```python
from build123d import *

# Parameters (mm, degrees)
F1_DEPTH = 45
F2_R     = 8.270702783
F2_R_2   = 7.5699344576
F2_R_3   = 0.4069488222
F3_DEPTH = 1.5


with BuildPart() as f1:
    # F0 (on Right) → F1 (new body)
    with BuildSketch(Plane.YZ):
        with BuildLine():
            Line((-22.4725382223, 23.5068366048), (0, 0))
            Line((0, 0), (12.3609593138, 0))
            ThreePointArc((12.3609593138, 0), (13.7751728762, 0.5857864376), (14.3609593138, 2))
            Line((14.3609593138, 2), (14.3609593138, 7))
            Line((14.3609593138, 7), (14.3609593138, 9))
            ThreePointArc((14.3609593138, 9), (14.068066095, 9.7071067812), (13.3609593138, 10))
            Line((13.3609593138, 10), (12.2823521785, 10))
            ThreePointArc((12.2823521785, 10), (11.5752453973, 9.7071067812), (11.2823521785, 9))
            Line((11.2823521785, 9), (11.2823521785, 7))
            ThreePointArc((11.2823521785, 7), (10.1107793032, 4.1715728753), (7.2823521785, 3))
            Line((7.2823521785, 3), (1.2823521785, 3))
            Line((1.2823521785, 3), (-25.4725382223, 30.9862840062))
            ThreePointArc((-25.4725382223, 30.9862840062), (-28.7578385809, 31.6975803479), (-30.6410287362, 28.913206851))
            Line((-30.6410287362, 28.913206851), (-30.6410287362, 0))
            Line((-30.6410287362, 0), (-27.6410287362, 0))
            Line((-27.6410287362, 0), (-27.6410287362, 21.4337594496))
            ThreePointArc((-27.6410287362, 21.4337594496), (-25.7578385809, 24.2181329465), (-22.4725382223, 23.5068366048))
        make_face()
    extrude(amount=F1_DEPTH)

    # F2 (on face) → F3 (cut)
    with BuildSketch(Plane(origin=(0, 2.1684905138, 2.0730771552), x_dir=(-1, 0, 0), z_dir=(0, 0.7228301713, 0.6910257184))):
        with Locations((-22.5, 20.6411760892)):
            Circle(F2_R)
        with Locations((-22.5, 20.6411760892)):
            Circle(F2_R_2, mode=Mode.SUBTRACT)
        with BuildLine():
            Line((-26.7460289363, 19.2989930163), (-26.7460289363, 21.0181410771))
            ThreePointArc((-26.7460289363, 21.0181410771), (-27.1604015057, 23.0993524994), (-27.5180879991, 21.0076531943))
            Line((-27.5180879991, 21.0076531943), (-27.5180879991, 19.1088523712))
            Line((-27.5180879991, 19.1088523712), (-27.3791737854, 18.8299436122))
            Line((-27.3791737854, 18.8299436122), (-27.1837860346, 18.5172446072))
            Line((-27.1837860346, 18.5172446072), (-26.9623473287, 18.2827226818))
            Line((-26.9623473287, 18.2827226818), (-26.68880485, 18.0481951684))
            Line((-26.68880485, 18.0481951684), (-26.3631585985, 17.8918484598))
            Line((-26.3631585985, 17.8918484598), (-25.9333048016, 17.7876148373))
            Line((-25.9333048016, 17.7876148373), (-18.7821220607, 17.7876148373))
            Line((-18.7821220607, 17.7876148373), (-18.5476560146, 17.8918484598))
            Line((-18.5476560146, 17.8918484598), (-18.3392427862, 18.0481951684))
            Line((-18.3392427862, 18.0481951684), (-18.0917512625, 18.2827226818))
            Line((-18.0917512625, 18.2827226818), (-17.9093908519, 18.5172446072))
            Line((-17.9093908519, 18.5172446072), (-17.7009776235, 18.8299436122))
            Line((-17.7009776235, 18.8299436122), (-17.5967700779, 19.1088523712))
            Line((-17.5967700779, 19.1088523712), (-17.5967700779, 21.0005989226))
            ThreePointArc((-17.5967700779, 21.0005989226), (-17.9118361845, 23.10197132), (-18.3392427862, 21.0205400333))
            Line((-18.3392427862, 21.0205400333), (-18.3392427862, 19.4162540138))
            Line((-18.3392427862, 19.4162540138), (-18.4043720365, 19.2468762398))
            Line((-18.4043720365, 19.2468762398), (-18.5606833547, 19.0123524517))
            Line((-18.5606833547, 19.0123524517), (-18.6909399927, 18.8429746777))
            Line((-18.6909399927, 18.8429746777), (-18.8602767885, 18.6866223812))
            Line((-18.8602767885, 18.6866223812), (-19.1989485174, 18.5302719474))
            Line((-19.1989485174, 18.5302719474), (-20.7229703665, 18.5302719474))
            Line((-20.7229703665, 18.5302719474), (-20.6578411162, 18.6735969037))
            Line((-20.6578411162, 18.6735969037), (-20.5836875976, 18.8169161692))
            Line((-20.5836875976, 18.8169161692), (-20.5836875976, 21.0127137605))
            ThreePointArc((-20.5836875976, 21.0127137605), (-21.0493362808, 23.0811417849), (-21.3742628694, 20.9859936039))
            Line((-21.3742628694, 20.9859936039), (-21.3742628694, 18.8429746777))
            Line((-21.3742628694, 18.8429746777), (-21.4133411646, 18.6866223812))
            Line((-21.4133411646, 18.6866223812), (-21.4784704149, 18.6084471643))
            Line((-21.4784704149, 18.6084471643), (-21.647805348, 18.5302719474))
            Line((-21.647805348, 18.5302719474), (-23.3281385154, 18.5302719474))
            Line((-23.3281385154, 18.5302719474), (-23.4714224935, 18.5693614185))
            Line((-23.4714224935, 18.5693614185), (-23.6147064716, 18.6735969037))
            Line((-23.6147064716, 18.6735969037), (-23.7134122117, 18.8038833277))
            Line((-23.7134122117, 18.8038833277), (-23.7134122117, 20.990443881))
            ThreePointArc((-23.7134122117, 20.990443881), (-24.0851049871, 23.0782021511), (-24.5004631579, 20.9986907413))
            Line((-24.5004631579, 20.9986907413), (-24.5004631579, 18.8038833439))
            Line((-24.5004631579, 18.8038833439), (-24.4874376804, 18.647538498))
            Line((-24.4874376804, 18.647538498), (-24.3441537023, 18.5172446072))
            Line((-24.3441537023, 18.5172446072), (-25.7248915732, 18.5172446072))
            Line((-25.7248915732, 18.5172446072), (-25.9463302791, 18.556330353))
            Line((-25.9463302791, 18.556330353), (-26.2198727578, 18.6996497214))
            Line((-26.2198727578, 18.6996497214), (-26.4282878488, 18.8560020179))
            Line((-26.4282878488, 18.8560020179), (-26.597622782, 19.0514381975))
            Line((-26.597622782, 19.0514381975), (-26.7460289363, 19.2989930163))
        make_face()
        with Locations((-27.1457448778, 22.0204138214)):
            Circle(F2_R_3, mode=Mode.SUBTRACT)
        with Locations((-24.0964107215, 21.9992231578)):
            Circle(F2_R_3, mode=Mode.SUBTRACT)
        with Locations((-21.0128873587, 22.0027193427)):
            Circle(F2_R_3, mode=Mode.SUBTRACT)
        with Locations((-17.9408062249, 22.0233220607)):
            Circle(F2_R_3, mode=Mode.SUBTRACT)
    extrude(amount=-F3_DEPTH, mode=Mode.SUBTRACT)


solid = f1.part
```
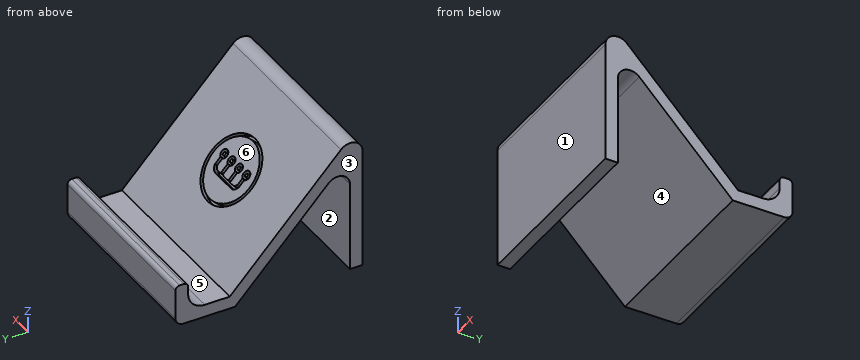
For this review, take the finished solid that the model builds, in its own axes (mm). Face numbers are marked on the shaded views. A direction names the side the tool comes from. Coordinates: 2 decimals unless noted, no trailing zeros. Order: outer loops, then holes, each group sorted by start corner. A loop starts at its lowest first (then second) coordinate and runs counter-clockwise, first axis right, second up. Notation, with made-up numbers: (42, 47.25) -> (92, 47.25) arc R30 cw to (92, 82.25) -> close; hole circle Ø4 at (-19, 38.5). An arc over 180 degrees is marked (long way). Answer as CSV lines item,"result".
Q1. Draft analysis for pull direction Y (two halves, no side actions). For the marked faces 1, 2 and 3, state which applies: released by +Y, released by -Y, zero draft, split by the parting line, or undercut.
Model answer:
face 1,"released by -Y"
face 2,"undercut"
face 3,"zero draft"
Q2. We need section C-C (y = 2). State the section outline as (x, z) points, plus the area to 3 significant figures.
Model answer:
outline,"(0, 0) -> (45, 0) -> (45, 3) -> (0, 3) -> close"
area,"135 mm2"
Q3. Wall thickness on line 1 along Y through (x, z) = (33.5, 8); line 2 along Y through (x, z) = (20.5, 8.5); line 3 along Y through (x, z) = (14, 22.5): over which ranges is each line inside the solid? List them lowest first. Write a range as [from, to].
Model answer:
line 1,"y = [-30.64, -27.64], [-7.65, -3.5], [11.28, 14.36]"
line 2,"y = [-30.64, -27.64], [-8.13, -3.98], [11.28, 14.36]"
line 3,"y = [-30.64, -27.45], [-21.51, -17.36]"
Q4. We need section A-A (z = 8). State the section outline as (x, y) points, plus the area to 3 significant figures.
Model answer:
outline,"(0, -30.64) -> (45, -30.64) -> (45, -27.64) -> (0, -27.64) -> close; (0, -7.65) -> (45, -7.65) -> (45, -3.5) -> (0, -3.5) -> close; (0, 11.28) -> (45, 11.28) -> (45, 14.36) -> (0, 14.36) -> close"
area,"460 mm2"
Q5. Clearance check with flat-ended pins moving along their axes: pin 1 Ø8 at (y, z) = (-1, 12) entering from +X; pin 2 Ø17 at (x, z) = (32.5, 12.5) entering from +Y; pin 3 Ø0.9 at (x, y) = (24.5, 13) entering from +Z; pin 4 Ø1.8 at (x, y) = (23, 4.5) entering from +Z. State where each tip first meets the part, or that it passes through.
Model answer:
pin 1,"passes through"
pin 2,"stops at y = 14.36"
pin 3,"stops at z = 10"
pin 4,"stops at z = 3"
Q6. We need section D-D (y = 9). State the section outline as (x, z) points, plus the area to 3 significant figures.
Model answer:
outline,"(0, 0) -> (45, 0) -> (45, 3.39) -> (0, 3.39) -> close"
area,"152 mm2"
Q7. We need section B-B (x = 12). State the section outline as (y, z) points, plus the area to 3 significant figures.
Model answer:
outline,"(-30.64, 0) -> (-27.64, 0) -> (-27.64, 21.43) arc R3 cw to (-22.47, 23.51) -> (0, 0) -> (12.36, 0) arc R2 ccw to (14.36, 2) -> (14.36, 9) arc R1 ccw to (13.36, 10) -> (12.28, 10) arc R1 ccw to (11.28, 9) -> (11.28, 7) arc R4 cw to (7.28, 3) -> (1.28, 3) -> (-25.47, 30.99) arc R3 ccw to (-30.64, 28.91) -> close"
area,"292 mm2"
Q8. For the marked faces 4, 5 and 6, list the 3-axis set-ups (+Z, -Z, +X, -X, +Y, -Y) from which the entire face can be reached by the end or side of a thin tool; tool diameter is ignored.
Model answer:
face 4,"-Z, +X, -X"
face 5,"+Z, +X, -X"
face 6,"+Z, +X, -X, +Y"
